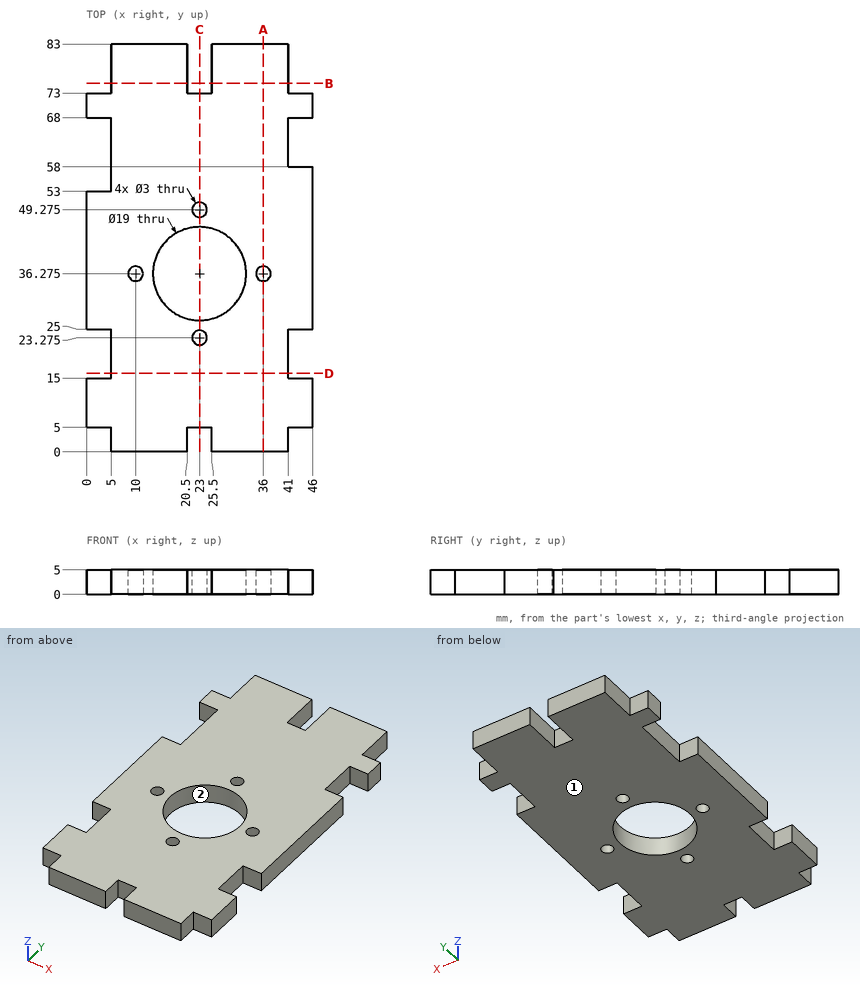
Study the drawing (mm; zero at the part's minimum x, y, z) and answer. Coordinates: 2 decimals unless noted, no trailing zeros. Write each loop counter-clockwise with the first axis right and the second up, starting at its lowest first coordinate (ties: lowest second). Pieces come first, ordered by that corner, then holes. Notation, with made-up numbers: (67.25, 11) - (85.25, 11) arc R28 cw to (85.25, 48) - close; hole circle Ø4 at (-3, 48). An arc over 180 degrees is marked (long way). One line per item, written item: value.
1) Each of these flat-tipped pins is pushed along its axis until it touches: pin 1 Ø2.5 at (y, z) = (76.5, 3.5) entering from +X; pin 2 Ø1.5 at (x, z) = (44.5, 2.5) entering from +Y. Where does it stop, or does it pass through?
Geometry check:
pin 1: stops at x = 41
pin 2: stops at y = 73
2) Consider line 1 along X through (y, z) = (36.5, 4.5); line 2 along Y through (x, z) = (23, 2.45) (3 decimals); line 3 along Y through (x, z) = (43, 1.2). Determine where each line is inside the solid, lowest interval first. Write a range as from..to.
Geometry check:
line 1: x = 0..8.52, 11.48..13.5, 32.5..34.52, 37.48..46
line 2: y = 5..21.775, 24.775..26.775, 45.775..47.775, 50.775..73
line 3: y = 5..15, 25..58, 68..73
3) Find section D-D (y = 16). Give the vertices of the cut face in (x, z).
Geometry check:
outline: (5, 0) - (41, 0) - (41, 5) - (5, 5) - close
4) For a pull along X with two mould halves and no side action, classify the marked faces 1 and 2 as pulls with the +X half, pulls with the -X half, needs draft (parallel to the pull), parting line crosses it, or undercut.
Geometry check:
face 1: needs draft
face 2: undercut
5) Find section B-B (y = 75). Give the vertices of the cut face in (x, z), and give its area (3 significant figures).
Geometry check:
outline: (5, 0) - (20.5, 0) - (20.5, 5) - (5, 5) - close; (25.5, 0) - (41, 0) - (41, 5) - (25.5, 5) - close
area: 155 mm2
6) Find section C-C (x = 23). Give the vertices of the cut face in (y, z) (3 decimals).
Geometry check:
outline: (5, 0) - (21.775, 0) - (21.775, 5) - (5, 5) - close; (24.775, 0) - (26.775, 0) - (26.775, 5) - (24.775, 5) - close; (45.775, 0) - (47.775, 0) - (47.775, 5) - (45.775, 5) - close; (50.775, 0) - (73, 0) - (73, 5) - (50.775, 5) - close
7) Find section A-A (x = 36). Give the vertices of the cut face in (y, z) (3 decimals), and give its area (3 significant figures).
Geometry check:
outline: (0, 0) - (34.775, 0) - (34.775, 5) - (0, 5) - close; (37.775, 0) - (83, 0) - (83, 5) - (37.775, 5) - close
area: 400 mm2
